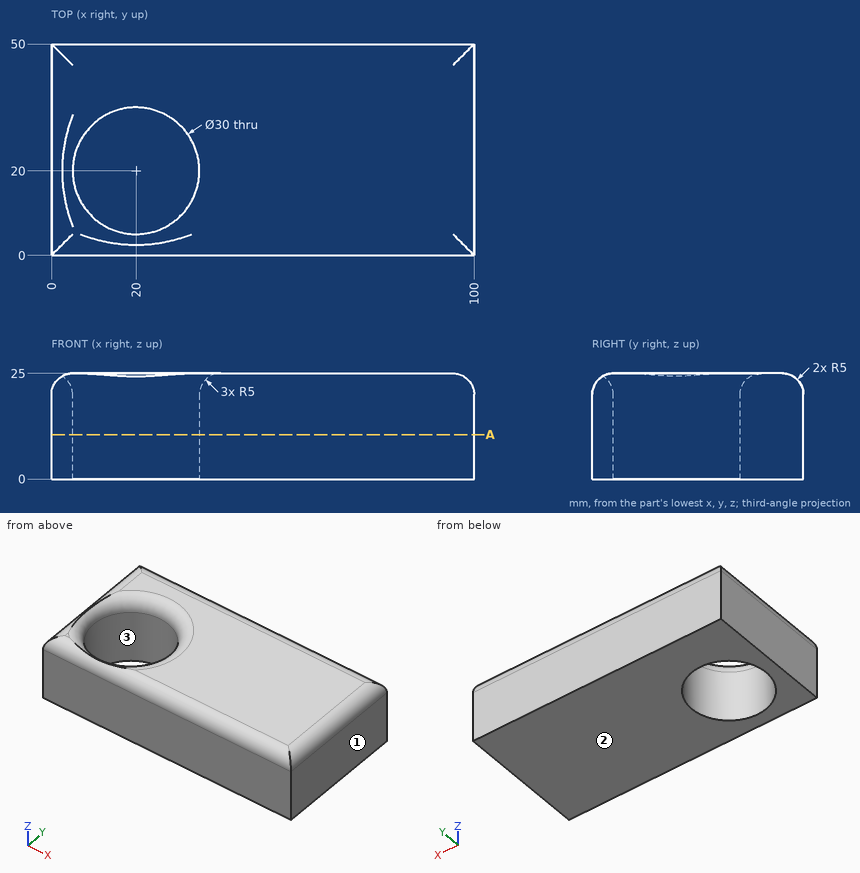
Geometry check sheet. Reference: drawing and pictorial views, mm from the part's lowest x, y, z. Round coordinates to 2 decimals unless told otherwise and drop trailing zeros. Loops run counter-clockwise (first coordinate to the right, second up) from the corner with the lowest first, then second, coordinate; pieces in that order, holes last. Notation, with made-up numbers: (55.5, 39) -> (94.5, 39) arc R18 ccw to (94.5, 49) -> close; hole circle Ø8 at (-21, 19). An arc over 180 degrees is marked (long way). Answer as a JSON object with one key per item and string values. Group by question number.
Item 1: Release check for a two-part mould opening along X. For the marked faces 1, 2 and 3 record: pulls with the +X half, pulls with the -X half, needs draft (parallel to the pull), parting line crosses it, or undercut.
Item 2: Thickness scan on line 1 along Y through (x, z) = (20, 6); line 2 along X through (y, z) = (23.5, 16.75); line 3 along Y through (x, z) = (24.5, 13.5). Record the ranges inside material, lowest first.
Item 3: Cross-section at A-A, the plane z = 10.5. Record the cut outline in (x, y), plus the area to 3 significant figures.
Determined:
{
 "1": {"face 1": "pulls with the +X half", "face 2": "needs draft", "face 3": "undercut"},
 "2": {"line 1": "y = 0 to 5, 35 to 50", "line 2": "x = 0 to 5.41, 34.59 to 100", "line 3": "y = 0 to 5.69, 34.31 to 50"},
 "3": {"outline": "(0, 0) -> (100, 0) -> (100, 50) -> (0, 50) -> close; hole circle Ø30 at (20, 20)", "area": "4,290 mm²"}
}
